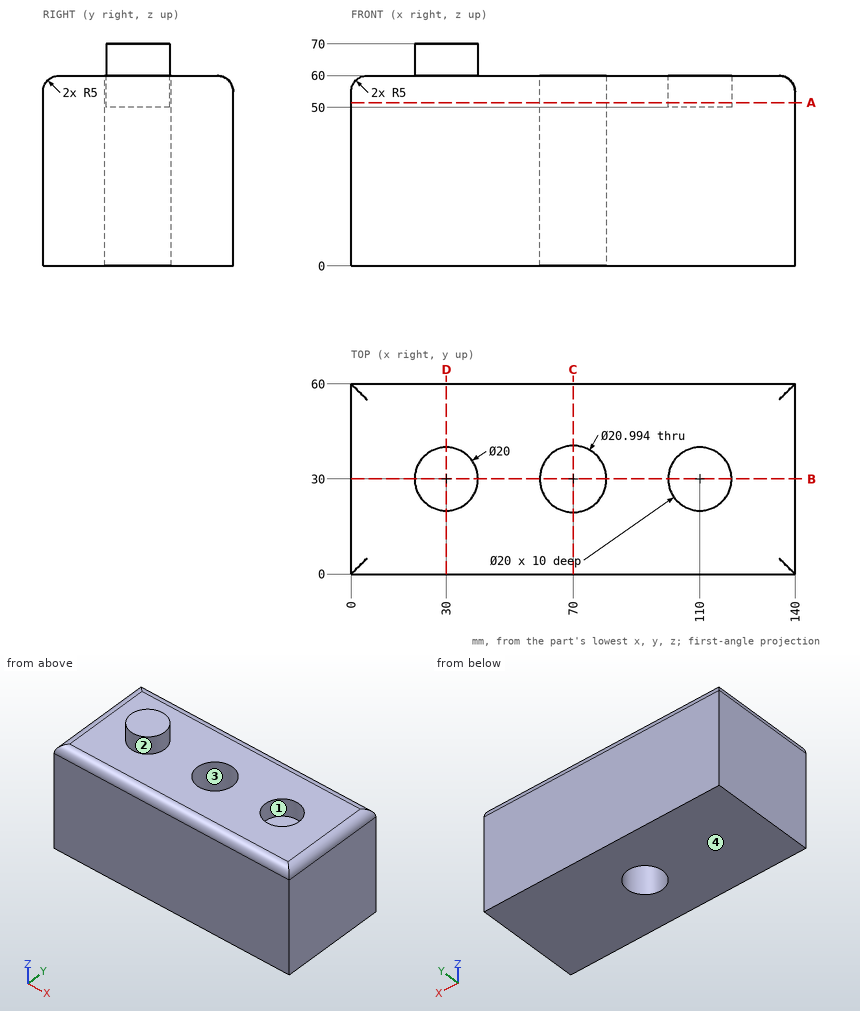
Answer from the drawing. Dimensions are ordinates in mm from the lowest x, y and z of the part. Coordinates: 2 decimals unless noted, no trailing zeros. Loops run counter-clockwise (first coordinate to the right, second up) from the corner with the lowest first, then second, coordinate; pieces in that order, holes last. Notation, with made-up numbers: (32, 14.5) -> (72, 14.5) arc R8 ccw to (72, 25.5) -> close; hole circle Ø8 at (26.25, 69). An arc over 180 degrees is marked (long way). Return JSON: item names as keys, results as strings.
Item 1: Find the intervals of material crossed by probe 1 along Y at (x, z) = (70, 36); probe 2 along Y at (x, z) = (110, 53.5); probe 3 along Z at (x, y) = (48.5, 24), in increasing order.
Answers:
{"probe 1": "y = 0 to 19.5, 40.5 to 60", "probe 2": "y = 0 to 20, 40 to 60", "probe 3": "z = 0 to 60"}
Item 2: Find section B-B (y = 30). Determine the outline of the cut face in (x, z), plus the area to 3 significant figures.
Answers:
{"outline": "(0, 0) -> (59.5, 0) -> (59.5, 60) -> (40, 60) -> (40, 70) -> (20, 70) -> (20, 60) -> (5, 60) arc R5 ccw to (0, 55) -> close; (80.5, 0) -> (140, 0) -> (140, 55) arc R5 ccw to (135, 60) -> (120, 60) -> (120, 50) -> (100, 50) -> (100, 60) -> (80.5, 60) -> close", "area": "7,130 mm2"}
Item 3: For a pull along X with two mould halves and no side action, classify the marked faces 1, 2, 3 and 4 as +X half, -X half, draft (parallel to the pull), parting line (faces both ways), or undercut.
Answers:
{"face 1": "undercut", "face 2": "parting line", "face 3": "undercut", "face 4": "draft"}
Item 4: Find section C-C (x = 70). Determine the outline of the cut face in (y, z), plus the area to 3 significant figures.
Answers:
{"outline": "(0, 0) -> (19.5, 0) -> (19.5, 60) -> (5, 60) arc R5 ccw to (0, 55) -> close; (40.5, 0) -> (60, 0) -> (60, 55) arc R5 ccw to (55, 60) -> (40.5, 60) -> close", "area": "2,330 mm2"}
Item 5: Flat-ended cylindrical pins translate along their axes: P1, Ø10, axis at y = 26.5, z = 52.5, coming from the -X side; P2, Ø16, axis at x = 110, y = 30, coming from the +Z side; P3, Ø15, axis at x = 86.5, y = 34.5, coming from the +Z side. Find the tip coordinate at first contact, or state that the pin passes through.
Answers:
{"P1": "stops at x = 0", "P2": "stops at z = 50", "P3": "stops at z = 60"}
Item 6: Find section A-A (z = 51.5). Determine the outline of the cut face in (x, y), plus the area to 3 significant figures.
Answers:
{"outline": "(0, 0) -> (140, 0) -> (140, 60) -> (0, 60) -> close; hole circle Ø20.99 at (70, 30); hole circle Ø20 at (110, 30)", "area": "7,740 mm2"}
Item 7: Find section D-D (x = 30). Determine the outline of the cut face in (y, z), plus the area to 3 significant figures.
Answers:
{"outline": "(0, 0) -> (60, 0) -> (60, 55) arc R5 ccw to (55, 60) -> (40, 60) -> (40, 70) -> (20, 70) -> (20, 60) -> (5, 60) arc R5 ccw to (0, 55) -> close", "area": "3,790 mm2"}
